```python
from build123d import *

# Parameters (mm, degrees)
BOSS_EXTRUDE1_START     = -8
BOSS_EXTRUDE1_OUTLINE_R = 1.1
BOSS_EXTRUDE1_DEPTH     = 8
SKETCH4_R               = 5.399616231
BOSS_EXTRUDE2_DEPTH     = 8
CUT_EXTRUDE1_DEPTH      = 12.881979778
CUT_EXTRUDE1_DEPTH_BACK = 12.881979778
SKETCH5_W               = 18.2
SKETCH5_H               = 5


# Read off the part's stored shape, not the designer's step: Boss-Extrude1
with BuildPart() as part:
    # Sketch1 → Revolve3 (revolve)
    with BuildSketch(Plane.XY):
        with BuildLine():
            Line((-5.399616231, -5.3975), (0, -5.3975))
            Line((0, -5.3975), (0, 2.6025))
            Line((0, 2.6025), (-3.988533565, 2.6025))
            ThreePointArc((-3.988533565, 2.6025), (-4.472061932, 1.637702149), (-4.725960888, 0.58881231))
            add(Edge.make_bspline(
                [(-4.725960888, 0.58881231), (-5.528679385, 0.558813228), (-5.399616231, 0.190451496), (-5.399616231, -0.666596714)],
                knots=[0, 0, 0, 0, 1, 1, 1, 1], degree=3))
            Line((-5.399616231, -0.666596714), (-5.399616231, -5.3975))
        make_face()
    revolve(axis=Axis((0, 8.574910523, 0), (0, -1, 0)))



with BuildPart() as body_2:
    # Boss-Extrude1 outline → Boss-Extrude1 (new body)
    # profile 1 of 2: a face of its own
    with BuildSketch(Plane.XZ.offset(5.3975).offset(BOSS_EXTRUDE1_START)):
        with BuildLine():
            add(Edge.make_bspline(
                [(6.6, -2.5), (5.362311666, -2.5), (4.636385799, -2.941104214), (3.959842535, -3.670899419)],
                knots=[0, 0, 0, 0, 1, 1, 1, 1], degree=3))
            ThreePointArc((6.6, -2.5), (9.1, 0), (6.6, 2.5))
            add(Edge.make_bspline(
                [(6.6, 2.5), (5.362311666, 2.5), (4.636385799, 2.941104214), (3.959842535, 3.670899419)],
                knots=[0, 0, 0, 0, 1, 1, 1, 1], degree=3))
            ThreePointArc((3.959842535, 3.670899419), (5.399616231, 0), (3.959842535, -3.670899419))
        make_face()
        with Locations((6.6, 0)):
            Circle(BOSS_EXTRUDE1_OUTLINE_R, mode=Mode.SUBTRACT)
    # profile 2 of 2: a face of its own
    with BuildSketch(Plane.XZ.offset(5.3975).offset(BOSS_EXTRUDE1_START)):
        with BuildLine():
            ThreePointArc((-6.6, 2.5), (-9.1, 0), (-6.6, -2.5))
            add(Edge.make_bspline(
                [(-6.6, -2.5), (-5.362311666, -2.5), (-4.636385799, -2.941104214), (-3.959842535, -3.670899419)],
                knots=[0, 0, 0, 0, 1, 1, 1, 1], degree=3))
            ThreePointArc((-3.959842535, -3.670899419), (-5.399616231, 0), (-3.959842535, 3.670899419))
            add(Edge.make_bspline(
                [(-6.6, 2.5), (-5.362311666, 2.5), (-4.636385799, 2.941104214), (-3.959842535, 3.670899419)],
                knots=[0, 0, 0, 0, 1, 1, 1, 1], degree=3))
        make_face()
        with Locations((-6.6, 0)):
            Circle(BOSS_EXTRUDE1_OUTLINE_R, mode=Mode.SUBTRACT)
    extrude(amount=BOSS_EXTRUDE1_DEPTH)


with BuildPart() as part_1:
    add(part.part)

    add(body_2.part)  # Boss-Extrude2 merges body 2
    # Sketch4 → Boss-Extrude2 (add)
    with BuildSketch(Plane.XZ.offset(5.3975)):
        Circle(SKETCH4_R)
    extrude(amount=-BOSS_EXTRUDE2_DEPTH)

    # Sketch5 → Cut-Extrude1 (cut, two sides: drawn at the far end of the back side and taken through both)
    with BuildSketch(Plane.XY.offset(-CUT_EXTRUDE1_DEPTH_BACK)):
        with Locations((0, 0.1025)):
            Rectangle(SKETCH5_W, SKETCH5_H)
    extrude(amount=CUT_EXTRUDE1_DEPTH + CUT_EXTRUDE1_DEPTH_BACK, mode=Mode.SUBTRACT)


solid = part_1.part
```
Here's how the part is built. I have some questions about the finished solid (model axes, mm). Round coordinates to 2 decimals unless told otherwise and drop trailing zeros. Loops run counter-clockwise (first coordinate to the right, second up) from the corner with the lowest first, then second, coordinate; pieces in that order, holes last.
1. Suppose I cut it at D-D, the plane z = 1.5. Please give me the cut outline in (x, y), and give its area (3 significant figures).
Answers:
outline: (-8.6, -5.4) - (8.6, -5.4) - (8.6, -2.4) - (-8.6, -2.4) - close
area: 51.6 mm2
2. Suppose I cut it at A-A, the plane z = 0. Please give me the cut outline in (x, y), and give its area (3 significant figures).
Answers:
outline: (-9.1, -5.4) - (-7.7, -5.4) - (-7.7, -2.4) - (-9.1, -2.4) - close; (-5.5, -5.4) - (5.5, -5.4) - (5.5, -2.4) - (-5.5, -2.4) - close; (7.7, -5.4) - (9.1, -5.4) - (9.1, -2.4) - (7.7, -2.4) - close
area: 41.4 mm2
3. Thinking about a two-plate mould opening in X: for faces 1 (the face through (9.1, -3.9, -0.1)), 2 (the face through (5.5, -3.9, 0)), 3 (the face through (-5.584, -3.876, -0.421)), 4 (the face through (0, -2.398, 0)), which applies, released by +X, released by -X, zero draft, split by the parting line, or undercut?
Answers:
face 1: released by +X
face 2: undercut
face 3: undercut
face 4: zero draft
4. Suppose I cut it at B-B, the plane x = 7. Please give me the cut outline in (y, z), and give its area (3 significant figures).
Answers:
outline: (-5.4, -2.47) - (-2.4, -2.47) - (-2.4, -1.02) - (-5.4, -1.02) - close; (-5.4, 1.02) - (-2.4, 1.02) - (-2.4, 2.47) - (-5.4, 2.47) - close
area: 8.66 mm2
5. Suppose I cut it at C-C, the plane y = -3.75. Give the number of separate pieces and of enclosed holes in the cut face, and give its area (3 significant figures).
Answers:
separate pieces: 1
enclosed holes: 2
area: 119 mm2
6. If I drill on probe 1 along X at (y, z) = (-3.45, 0); probe 2 along Z at (x, y) = (-6.6, -4.6); probe 3 along X at (y, z) = (-3, -1), over which ranges is the centre line in solid material (lowest first)?
Answers:
probe 1: x = -9.1 to -7.7, -5.5 to 5.5, 7.7 to 9.1
probe 2: z = -2.5 to -1.1, 1.1 to 2.5
probe 3: x = -8.89 to -7.06, -6.14 to 6.14, 7.06 to 8.89
7. Will this pin go through, and if not, where does the flat tip stop? pin 1 (1.8 mm diameter, centred on x = -6.6, z = 0, fed in from -Y).
Answers:
pin 1: passes through
